Could you check a few things on this model? Use its own coordinates, in mm. Face numbers are marked on the shaded views. A direction names the side the tool comes from. Coordinates: 2 decimals unless noted, no trailing zeros. Loops run counter-clockwise (first coordinate to the right, second up) from the corner with the lowest first, then second, coordinate; pieces in that order, holes last. Notation, with made-up numbers: M 87,-1 L 130,-1 A30 ccw 130,24 Z; hole C 3.5,28.25 d8. An arc over 180 degrees is marked long. Use one line per item in the form item = value. Start each with the question number.
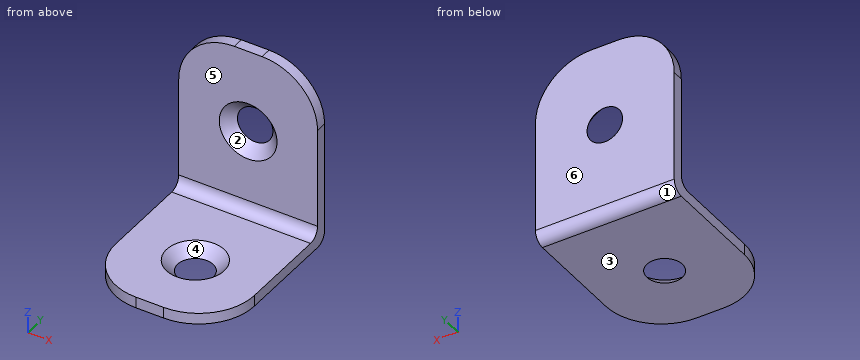
```python
from build123d import *

# Parameters (mm, degrees)
EXTRUDE_1_DEPTH = 2
EXTRUDE_2_DEPTH = 2
FILLET_1_R      = 2
FILLET_2_R      = 2


with BuildPart() as part:
    # Эскиз1 → Бобышка-Вытянуть1 (new body)
    with BuildSketch(Plane(origin=(0, 0, 0), x_dir=(1, 0, 0), z_dir=(0, 1, 0))):
        with BuildLine():
            Line((-2.5, -15), (2.5, -15))
            ThreePointArc((2.5, -15), (9.571067812, -12.071067812), (12.5, -5))
            Line((12.5, -5), (12.5, 15))
            Line((12.5, 15), (-12.5, 15))
            Line((-12.5, 15), (-12.5, -5))
            ThreePointArc((-12.5, -5), (-9.571067812, -12.071067812), (-2.5, -15))
        make_face()
    extrude(amount=EXTRUDE_1_DEPTH)

    # Эскиз3 → Бобышка-Вытянуть2 (add)
    with BuildSketch(Plane(origin=(0, 0, -15), x_dir=(-1, 0, 0), z_dir=(0, 0, -1))):
        with BuildLine():
            Line((-2.5, -28), (2.5, -28))
            ThreePointArc((2.5, -28), (9.571067812, -25.071067812), (12.5, -18))
            Line((12.5, -18), (12.5, 2))
            Line((12.5, 2), (-12.5, 2))
            Line((-12.5, 2), (-12.5, -18))
            ThreePointArc((-12.5, -18), (-9.571067812, -25.071067812), (-2.5, -28))
        make_face()
    extrude(amount=EXTRUDE_2_DEPTH)

    # Скругление1
    fillet_1_edges = [part.edges().sort_by_distance(p)[0] for p in [
        (0, 0, -15),
    ]]
    fillet(fillet_1_edges, radius=FILLET_1_R)

    # Скругление2
    fillet_2_edges = [part.edges().sort_by_distance(p)[0] for p in [
        (0, 2, -17),
    ]]
    fillet(fillet_2_edges, radius=FILLET_2_R)

    # Эскиз7 → Зенковка для винта с полупотайной головкой M52 (revolve, cut)
    with BuildSketch(Plane(origin=(0, -15.034247801, -15), x_dir=(0, -1, 0), z_dir=(1, 0, 0))):
        Polygon((0, 0), (0, 2), (2.75, 2), (2.75, 2.45), (5.2, 0), align=None)
    revolve(axis=Axis((0, -15.034247801, -8.65), (0, 0, -1)), mode=Mode.SUBTRACT)

    # Эскиз9 → Зенковка для винта с полупотайной головкой M53 (revolve, cut)
    with BuildSketch(Plane(origin=(0, 0, 0), x_dir=(0, 0, -1), z_dir=(1, 0, 0))):
        Polygon((0, 0), (0, 2), (2.75, 2), (2.75, 2.45), (5.2, 0), align=None)
    revolve(axis=Axis((0, -6.35, 0), (0, 1, 0)), mode=Mode.SUBTRACT)


solid = part.part
```
Item 1: I want a section at B-B (x = 0). Write out the boundary of the cut face in (y, z).
Item 2: I want a section at D-D (y = -3.5). Write out the boundary of the cut face in (x, z).
Item 3: Thinking about a two-plate mould opening in Y: for the marked faces 1, 2, 3 and 4, which applies, pulls with the +Y half, pulls with the -Y half, needs draft (parallel to the pull), parting line crosses it, or undercut?
Item 4: For the marked faces 5 and 6, which set-ups out of +Z, -Z, +X, -X, +Y, -Y let a thin tool reach every point of the face, with its end or its side?
Item 5: I want a section at C-C (x = -7.5). Write out the boundary of the cut face in (y, z).
Item 6: I want a section at A-A (z = 0). Write out the boundary of the cut face in (x, y), plus the area to 3 significant figures.
Item 7: Please list where these lines run through material, in increasing order: line 1 along Y through (x, z) = (-6.25, 10); line 2 along Z through (x, y) = (-4.75, -12.5); line 3 along X through (y, z) = (0.5, 8.5).
Item 8: I'm going to push flat-ended pins straight in: P1, Ø5, axis at x = -7, z = 6.5, coming from the -Y side; P2, Ø12.5, axis at x = 5, y = -13.5, coming from the +Z side; P3, Ø8, axis at y = -16.5, z = -7.5, coming from the +X side. Where does each tip first touch, or does it pass through?
Worked answers:
q1.outline = M -28,-17 L -18.23,-17 L -20.23,-15 L -28,-15 Z; M -11.83,-17 L 0,-17 A2 ccw 2,-15 L 2,-3.2 L 0,-5.2 L 0,-13 A2 cw -2,-15 L -9.83,-15 Z; M 0,5.2 L 2,3.2 L 2,15 L 0,15 Z
q2.outline = M -12.5,-17 L 12.5,-17 L 12.5,-15 L -12.5,-15 Z
q3.face_1 = pulls with the +Y half
q3.face_2 = pulls with the -Y half
q3.face_3 = needs draft
q3.face_4 = undercut
q4.face_5 = +Z, +X, -X, -Y
q4.face_6 = +Z, -Z, +X, -X, +Y
q5.outline = M -26.66,-17 L 0,-17 A2 ccw 2,-15 L 2,13.66 L 0,13.66 L 0,-13 A2 cw -2,-15 L -26.66,-15 Z
q6.outline = M -12.5,0 L -5.2,0 L -3.2,2 L -12.5,2 Z; M 3.2,2 L 5.2,0 L 12.5,0 L 12.5,2 Z
q6.area = 33.2 mm²
q7.line_1 = 0 to 2
q7.line_2 = -17 to -15
q7.line_3 = -11.87 to 11.87
q8.P1 = 0
q8.P2 = -15
q8.P3 = through
